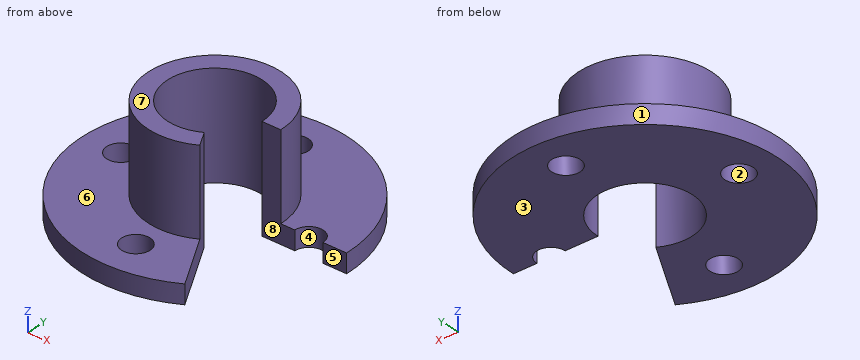
```python
from build123d import *

# Parameters (mm, degrees)
F1_ANGLE = 300
F2_R     = 7.5
F3_DEPTH = 10.001


with BuildPart() as f1:
    # F0 (on Front) → F1 (revolve)
    with BuildSketch(Plane.XZ):
        Polygon((35, 55), (25, 55), (25, 0), (70, 0), (70, 10), (35, 10), align=None)
    revolve(axis=Axis((0, 0, 30.149998), (0, 0, 1)), revolution_arc=F1_ANGLE)

    # F2 (on face) → F3 (cut, through all)
    with BuildSketch(Plane.XY.offset(10)):
        with BuildLine():
            Line((42.465329, 0), (57.465329, 0))
            ThreePointArc((57.465329, 0), (49.965329, 7.5), (42.465329, 0))
        make_face()
        with Locations((0, 49.965329)):
            Circle(F2_R)
        with Locations((-49.965329, 0)):
            Circle(F2_R)
        with Locations((0, -49.965329)):
            Circle(F2_R)
    extrude(amount=-F3_DEPTH, mode=Mode.SUBTRACT)


solid = f1.part
```
For this review, take the finished solid that the model builds, in its own axes (mm). Face numbers are marked on the shaded views. A direction names the side the tool comes from. Give positions to 0.01 mm unless a question says otherwise; leave off trailing zeros. Write each loop counter-clockwise with the first axis right and the second up, starting at its lowest first coordinate (ties: lowest second). Pieces come first, ordered by that corner, then holes. Notation, with made-up numbers: M -2.75,28 L 48.25,28 A19 ccw 48.25,54 Z; hole C 19,61 d7. An arc over 180 degrees is marked long. Answer as CSV lines item,"result".
1. Consider section C-C, the plane z = 21. Write out the cut boundary in (x, y), then the cut area to 3 significant figures.
Findings:
outline,"M 12.5,-21.65 A25 cw long 25,0 L 35,0 A35 ccw long 17.5,-30.31 Z"
area,"1,570 mm2"
2. For pin 1 (10 mm diameter, centred on y = 23, z = 19, fed in from +X); pin 2 (10 mm diameter, centred on x = 34.5, y = 28.5, fed in from +Z); pin 3 (4 mm diameter, centred on y = -32.5, z = 31.5, fed in from +X); pin 4 (13.5 mm diameter, centred on x = -49.97, y = 0, fed in from +Z), all flat-tipped, find the tip position at first contact; note any pin that passes through.
Findings:
pin 1,"stops at x = 30.02"
pin 2,"stops at z = 10"
pin 3,"stops at x = 17.17"
pin 4,"passes through"
3. Wall thickness on line 1 (Y direction, x = 0, z = 2.25); line 2 (Z direction, x = -31, y = -56.5); line 3 (Y direction, x = 31.5, z = 9): over which ranges is each line inside the solid? List them lowest first.
Findings:
line 1,"y = -70 to -57.47, -42.47 to -25, 25 to 42.47, 57.47 to 70"
line 2,"z = 0 to 10"
line 3,"y = -62.51 to -54.56, 0 to 62.51"
4. Draft analysis for pull direction X (two halves, no side actions). For the marked faces 1, 2 and 3, state which applies: +X half, -X half, draft (parallel to the pull), parting line (faces both ways), or undercut.
Findings:
face 1,"parting line"
face 2,"undercut"
face 3,"draft"
5. Consider section A-A, the plane x = 0. Write out the cut boundary in (y, z), then the cut area to 3 significant figures.
Findings:
outline,"M -70,0 L -57.47,0 L -57.47,10 L -70,10 Z; M -42.47,0 L -25,0 L -25,55 L -35,55 L -35,10 L -42.47,10 Z; M 25,0 L 42.47,0 L 42.47,10 L 35,10 L 35,55 L 25,55 Z; M 57.47,0 L 70,0 L 70,10 L 57.47,10 Z"
area,"1,500 mm2"
6. Consider section D-D, the plane y = 61.5. Write out the cut boundary in (x, z).
Findings:
outline,"M -33.43,0 L 33.43,0 L 33.43,10 L -33.43,10 Z"
7. Consider section B-B, the plane y = -2.5. Write out the cut boundary in (x, z), then the cut area to 3 significant figures.
Findings:
outline,"M -69.96,0 L -57.04,0 L -57.04,10 L -69.96,10 Z; M -42.89,0 L -24.87,0 L -24.87,55 L -34.91,55 L -34.91,10 L -42.89,10 Z"
area,"761 mm2"
8. For the marked faces 4, 5, 6, 7 and 8, list the 3-axis set-ups (+Z, -Z, +X, -X, +Y, -Y) from which the entire face can be reached by the end or side of a thin tool; tool diameter is ignored.
Findings:
face 4,"+Z, -Z, -Y"
face 5,"+Z, -Z, +X, -Y"
face 6,"+Z"
face 7,"+Z, +X, -X, +Y, -Y"
face 8,"+Z, -Z, +X"
